CAD build for the part. Positions are in the model's coordinates, mm. Face numbers are marked on the shaded views. A direction names the side the tool comes from. Round coordinates to 2 decimals unless told otherwise and drop trailing zeros. Write each loop counter-clockwise with the first axis right and the second up, starting at its lowest first coordinate (ties: lowest second). Pieces come first, ordered by that corner, then holes. Notation, with made-up numbers: (67, 48.25) -> (81, 48.25) arc R18 cw to (81, 71.25) -> close; hole circle Ø4 at (19, -6.75). An arc over 180 degrees is marked (long way). Put each result on its own line as item: value. Start each with the question number.
1. Drill centre lines: line 1 (Z direction, x = 36, y = 3); line 2 (Z direction, x = 5.2, y = 16); line 3 (Y direction, x = 16, z = 0.85). Where is each one in solid material? Low to high. Write a range as from..to.
2. Pull direction Y, two halves, no side cores. Call the marked faces 1, 2, 3 and 4: pulls with the +Y half, pulls with the -Y half, needs draft (parallel to the pull), parting line crosses it, or undercut.
3. Saw through at D-D on z = 21. List the corners of the cut face in (x, y).
4. Saw through at A-A on y = 56. List the corners of the cut face in (x, z), and give its area (3 significant figures).
5. Flat gauge pins, fed straight in: P1, Ø4.5, axis at x = 15, z = 49, coming from the +Y side; P2, Ø2, axis at x = 23, z = 50, coming from the +Y side; P3, Ø2, axis at x = 34.5, z = 15.5, coming from the -Y side. Where does each tip first touch, or does it go through?
6. Saw through at C-C on z = 56. State how many separate pieces and enclosed holes the cut face has, and give its area (3 significant figures).
7. 3-axis set-ups, long thin cutter, end or side, ignore diameter. For the marked faces 5, 6 and 7: which of +Z, -Z, +X, -X, +Y, -Y reach the whole face in a straight line?
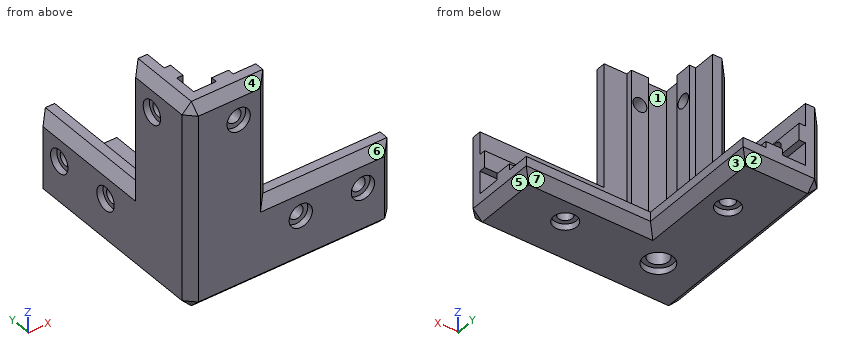
from build123d import *

# Parameters (mm, degrees)
F1_DEPTH  = 6
F3_DEPTH  = 20
F5_DEPTH  = 40
F7_DEPTH  = 60
F9_DEPTH  = 2
F11_DEPTH = 2
F13_DEPTH = 2
F14_R     = 2.25
F15_DEPTH = 8
F16_R     = 2.25
F17_DEPTH = 8
F18_R     = 3.25
F18_R_2   = 2.25
F19_DEPTH = 8.001
F20_R     = 3.75
F21_DEPTH = 2
F22_R     = 3.75
F23_DEPTH = 2
F24_R     = 3.75
F24_R_2   = 4.75
F25_DEPTH = 2
F26_SIZE  = 3


with BuildPart() as f1:
    # F0 (on Top) → F1 (new body)
    with BuildSketch(Plane.XY):
        Polygon((0, 66), (0, 0), (66, 0), (66, 26), (26, 26), (26, 66), align=None)
    extrude(amount=F1_DEPTH)

    # F2 (on face) → F3 (join)
    with BuildSketch(Plane.XY.offset(6)):
        Polygon((6, 66), (0, 66), (0, 0), (66, 0), (66, 6), (6, 6), align=None)
    extrude(amount=F3_DEPTH)

    # F4 (on face) → F5 (join)
    with BuildSketch(Plane.XY.offset(26)):
        Polygon((6, 6), (6, 26), (0, 26), (0, 0), (26, 0), (26, 6), align=None)
    extrude(amount=F5_DEPTH)

    # F6 (on face) → F7 (join)
    with BuildSketch(Plane.XY.offset(6)):
        Polygon((13.29, 6), (16, 6), (18.71, 6), (18.71, 8), (13.29, 8), align=None)
        Polygon((6, 18.71), (6, 16), (6, 13.29), (8, 13.29), (8, 18.71), align=None)
    extrude(amount=F7_DEPTH)

    # F8 (on face) → F9 (join)
    with BuildSketch(Plane.XY.offset(6)):
        Polygon((66, 13.29), (66, 16), (66, 18.71), (26, 18.71), (26, 13.29), align=None)
        Polygon((18.71, 66), (16, 66), (13.29, 66), (13.29, 26), (18.71, 26), align=None)
    extrude(amount=F9_DEPTH)

    # F10 (on face) → F11 (join)
    with BuildSketch(Plane(origin=(0, 6, 0), x_dir=(-1, 0, 0), z_dir=(0, 1, 0))):
        Polygon((-66, 18.71), (-66, 16), (-66, 13.29), (-26, 13.29), (-26, 16), (-26, 18.71), align=None)
    extrude(amount=F11_DEPTH)

    # F12 (on face) → F13 (join)
    with BuildSketch(Plane.YZ.offset(6)):
        Polygon((66, 13.29), (66, 16), (66, 18.71), (26, 18.71), (26, 13.29), align=None)
    extrude(amount=F13_DEPTH)

    # F14 (on face) → F15 (cut, through all)
    with BuildSketch(Plane.XZ):
        with Locations((56, 16)):
            Circle(F14_R)
        with Locations((16, 56)):
            Circle(F14_R)
        with Locations((36, 16)):
            Circle(F14_R)
    extrude(amount=-F15_DEPTH, mode=Mode.SUBTRACT)

    # F16 (on face) → F17 (cut, through all)
    with BuildSketch(Plane(origin=(0, 0, 0), x_dir=(0, -1, 0), z_dir=(-1, 0, 0))):
        with Locations((-16, 56)):
            Circle(F16_R)
        with Locations((-56, 16)):
            Circle(F16_R)
        with Locations((-36, 16)):
            Circle(F16_R)
    extrude(amount=-F17_DEPTH, mode=Mode.SUBTRACT)

    # F18 (on face) → F19 (cut, through all)
    with BuildSketch(Plane(origin=(0, 0, 0), x_dir=(1, 0, 0), z_dir=(0, 0, -1))):
        with Locations((16, -16)):
            Circle(F18_R)
        with Locations((46, -16)):
            Circle(F18_R_2)
        with Locations((16, -46)):
            Circle(F18_R_2)
    extrude(amount=-F19_DEPTH, mode=Mode.SUBTRACT)

    # F20 (on face) → F21 (cut)
    with BuildSketch(Plane.XZ):
        with Locations((16, 56)):
            Circle(F20_R)
        with Locations((36, 16)):
            Circle(F20_R)
        with Locations((56, 16)):
            Circle(F20_R)
    extrude(amount=-F21_DEPTH, mode=Mode.SUBTRACT)

    # F22 (on face) → F23 (cut)
    with BuildSketch(Plane(origin=(0, 0, 0), x_dir=(0, -1, 0), z_dir=(-1, 0, 0))):
        with Locations((-16, 56)):
            Circle(F22_R)
        with Locations((-36, 16)):
            Circle(F22_R)
        with Locations((-56, 16)):
            Circle(F22_R)
    extrude(amount=-F23_DEPTH, mode=Mode.SUBTRACT)

    # F24 (on face) → F25 (cut)
    with BuildSketch(Plane(origin=(0, 0, 0), x_dir=(1, 0, 0), z_dir=(0, 0, -1))):
        with Locations((16, -46)):
            Circle(F24_R)
        with Locations((16, -16)):
            Circle(F24_R_2)
        with Locations((46, -16)):
            Circle(F24_R)
    extrude(amount=-F25_DEPTH, mode=Mode.SUBTRACT)

    # F26
    f26_edges = [f1.edges().sort_by_distance(p)[0] for p in [
        (33, 0, 0),
        (0, 33, 0),
        (0, 0, 33),
        (0, 26, 46),
        (0, 46, 26),
        (26, 0, 46),
        (46, 0, 26),
        (0, 13, 66),
        (13, 0, 66),
        (0, 66, 13),
        (13, 66, 0),
        (66, 0, 13),
        (66, 13, 0),
        (46, 26, 0),
        (26, 46, 0),
    ]]
    chamfer(f26_edges, length=F26_SIZE)


solid = f1.part
Return value:
1. line 1: z = 0..13.75, 18.25..26
1. line 2: z = 0..53.75, 58.25..66
1. line 3: y = 2.15..11.25, 20.75..42.25, 49.75..63.85
2. face 1: undercut
2. face 2: pulls with the +Y half
2. face 3: needs draft
2. face 4: pulls with the -Y half
3. outline: (0, 3) -> (3, 0) -> (63, 0) -> (66, 3) -> (66, 6) -> (18.71, 6) -> (18.71, 8) -> (13.29, 8) -> (13.29, 6) -> (6, 6) -> (6, 13.29) -> (8, 13.29) -> (8, 18.71) -> (6, 18.71) -> (6, 66) -> (3, 66) -> (0, 63) -> close
4. outline: (0, 3) -> (3, 0) -> (23, 0) -> (26, 3) -> (26, 6) -> (18.71, 6) -> (18.71, 8) -> (13.29, 8) -> (13.29, 6) -> (6, 6) -> (6, 13.29) -> (8, 13.29) -> (8, 13.75) -> (2, 13.75) -> (2, 12.25) -> (0, 12.25) -> close; (0, 19.75) -> (2, 19.75) -> (2, 18.25) -> (8, 18.25) -> (8, 18.71) -> (6, 18.71) -> (6, 26) -> (3, 26) -> (0, 23) -> close
4. area: 242 mm^2
5. P1: stops at y = 8
5. P2: stops at y = 6
5. P3: stops at y = 2
6. separate pieces: 3
6. enclosed holes: 0
6. area: 200 mm^2
7. face 5: -Z, +X, +Y, -Y
7. face 6: +Z, +X, -Y
7. face 7: -Z, +X, +Y
